Input: part model. Units: mm. Frame: model coordinates. Give positions to 0.01 mm unless a question says otherwise; leave off trailing zeros. Order: outer loops, then holes, each group sorted by start corner. A loop starts at its lowest first (then second) coordinate and runs counter-clockwise, first axis right, second up. Notation, with made-up numbers: (23.25, 57.25) - (59.25, 57.25) arc R31 ccw to (59.25, 94.25) - close; hole circle Ø8 at (5, 19). An arc over 180 degrees is marked (long way). Answer in a Markdown table with one row per item. Add a question column.
1. Ray query, line 1 (Z direction, x = -90.5, y = 2.7); line 2 (X direction, y = 2.1, z = 195); line 3 (Z direction, x = -74.5, y = 2.8). Return the intervals inside material, ascending. Write a range as [from, to].
2. Section query B-B on x = -109. Return loops of the section in (y, z) (3 decimals), and give its area (4 significant figures).
3. Contact query for flat-ended pins moving along their axis: pin 1 (2.5 mm diameter, centred on x = 39.5, z = -16.5, fed in from +Y); pin 2 (1 mm diameter, centred on y = 1, z = 45, fed in from -X); pin 3 (1.2 mm diameter, centred on x = -126.5, y = 1.5, fed in from +Z); pin 4 (1 mm diameter, centred on x = 36.5, z = 103.5, fed in from -Y). Output: stop coordinate, or through.
4. Section query C-C on x = -44. Return loops of the section in (y, z) (3 decimals).
5. Section query A-A on z = 195. Return loops of the section in (x, y).
6. Section query D-D on y = 1.9. Count the separate pieces of the cut face and the enclosed holes in it, and give its area (3 significant figures).
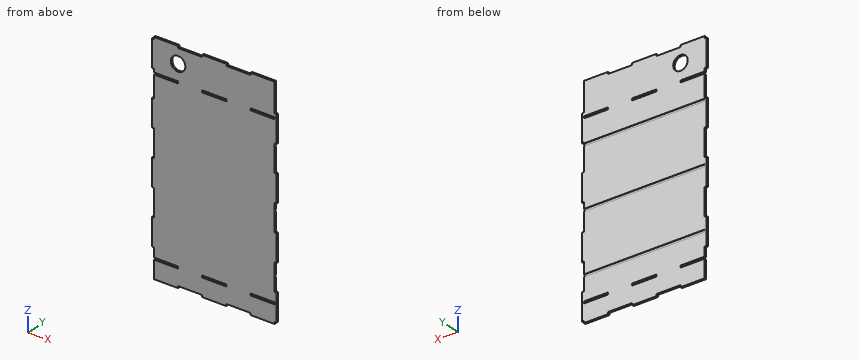
Autodesk Inventor part; units mm, degrees
ref_plane "YZ Plane" through (0, 0, 0) normal (1, 0, 0) x (0, 1, 0)
ref_plane "XZ Plane" through (0, 0, 0) normal (0, 1, 0) x (-1, 0, 0)
ref_plane "XY Plane" through (0, 0, 0) normal (0, 0, 1) x (1, 0, 0)
sketch "Sketch1" plane through (0, 0, 0) normal (0, 1, 0) x (-1, 0, 0)
  line L0 (-125, 225) -> (125, 225) construction
  line L1 (125, 225) -> (125, -225) construction
  line L2 (125, -225) -> (-125, -225) construction
  line L3 (-125, -225) -> (-125, 225) construction
  line L4 (-125, 225) -> (125, -225) construction
  line L5 (125, 225) -> (-125, -225) construction
  line L6 (125, 225) -> (75, 225) construction
  line L7 (75, 225) -> (75, 229)
  line L8 (75, 229) -> (125, 229)
  line L9 (125, 229) -> (125, 225)
  line L10 (125, 225) -> (129, 225)
  line L11 (129, 225) -> (129, 168.75)
  line L12 (129, 168.75) -> (125, 168.75)
  line L13 (125, 168.75) -> (125, 225) construction
  line L14 (-125, 225) -> (-129, 225) construction
  line L15 (-129, 225) -> (-129, 168.75) construction
  line L16 (-129, 168.75) -> (-125, 168.75)
  line L17 (-125, 168.75) -> (-125, 225)
  line L18 (125, -225) -> (75, -225) construction
  line L19 (75, -225) -> (75, -229)
  line L20 (75, -229) -> (125, -229)
  line L21 (125, -229) -> (125, -225)
  line L22 (125, 112.5) -> (125, 168.75)
  line L23 (125, 168.75) -> (129, 168.75)
  line L24 (129, 112.5) -> (125, 112.5)
  line L25 (129, 168.75) -> (129, 112.5) construction
  line L26 (-125, 112.5) -> (-125, 168.75) construction
  line L27 (-125, 168.75) -> (-129, 168.75)
  line L28 (-129, 168.75) -> (-129, 112.5)
  line L29 (-129, 112.5) -> (-125, 112.5)
  line L30 (125, 56.25) -> (125, 112.5) construction
  line L31 (125, 112.5) -> (129, 112.5)
  line L32 (129, 56.25) -> (125, 56.25)
  line L33 (129, 112.5) -> (129, 56.25)
  line L34 (-125, 56.25) -> (-125, 112.5)
  line L35 (-125, 112.5) -> (-129, 112.5)
  line L36 (-129, 112.5) -> (-129, 56.25) construction
  line L37 (-129, 56.25) -> (-125, 56.25)
  line L38 (125, 0) -> (125, 56.25)
  line L39 (125, 56.25) -> (129, 56.25)
  line L40 (129, 0) -> (125, 0)
  line L41 (129, 56.25) -> (129, 0) construction
  line L42 (-125, 0) -> (-125, 56.25) construction
  line L43 (-125, 56.25) -> (-129, 56.25)
  line L44 (-129, 56.25) -> (-129, 0)
  line L45 (-129, 0) -> (-125, 0)
  line L46 (125, -56.25) -> (125, 0) construction
  line L47 (125, 0) -> (129, 0)
  line L48 (129, -56.25) -> (125, -56.25)
  line L49 (129, 0) -> (129, -56.25)
  line L50 (-125, -56.25) -> (-125, 0)
  line L51 (-125, 0) -> (-129, 0)
  line L52 (-129, 0) -> (-129, -56.25) construction
  line L53 (-129, -56.25) -> (-125, -56.25)
  line L54 (125, -112.5) -> (125, -56.25)
  line L55 (125, -56.25) -> (129, -56.25)
  line L56 (129, -112.5) -> (125, -112.5)
  line L57 (129, -56.25) -> (129, -112.5) construction
  line L58 (-125, -112.5) -> (-125, -56.25) construction
  line L59 (-125, -56.25) -> (-129, -56.25)
  line L60 (-129, -56.25) -> (-129, -112.5)
  line L61 (-129, -112.5) -> (-125, -112.5)
  line L62 (125, -168.75) -> (125, -112.5) construction
  line L63 (125, -112.5) -> (129, -112.5)
  line L64 (129, -168.75) -> (125, -168.75)
  line L65 (129, -112.5) -> (129, -168.75)
  line L66 (-125, -168.75) -> (-125, -112.5)
  line L67 (-125, -112.5) -> (-129, -112.5)
  line L68 (-129, -112.5) -> (-129, -168.75) construction
  line L69 (-129, -168.75) -> (-125, -168.75)
  line L70 (125, -225) -> (125, -168.75)
  line L71 (125, -168.75) -> (129, -168.75)
  line L72 (129, -225) -> (125, -225) construction
  line L73 (129, -168.75) -> (129, -225) construction
  line L74 (-125, -225) -> (-125, -168.75) construction
  line L75 (-125, -168.75) -> (-129, -168.75)
  line L76 (-129, -168.75) -> (-129, -225)
  line L77 (-129, -225) -> (-125, -225)
  line L78 (75, 229) -> (75, 225)
  line L79 (25, 225) -> (25, 229)
  line L80 (25, 229) -> (75, 229) construction
  line L81 (75, 225) -> (25, 225)
  line L82 (75, -225) -> (25, -225)
  line L83 (25, -225) -> (25, -229)
  line L84 (25, -229) -> (75, -229) construction
  line L85 (75, -229) -> (75, -225)
  line L86 (25, 229) -> (25, 225)
  line L87 (-25, 225) -> (-25, 229)
  line L88 (-25, 229) -> (25, 229)
  line L89 (25, 225) -> (-25, 225) construction
  line L90 (25, -225) -> (-25, -225) construction
  line L91 (-25, -225) -> (-25, -229)
  line L92 (-25, -229) -> (25, -229)
  line L93 (25, -229) -> (25, -225)
  line L94 (-25, 229) -> (-25, 225)
  line L95 (-75, 225) -> (-75, 229)
  line L96 (-75, 229) -> (-25, 229) construction
  line L97 (-25, 225) -> (-75, 225)
  line L98 (-25, -225) -> (-75, -225)
  line L99 (-75, -225) -> (-75, -229)
  line L100 (-75, -229) -> (-25, -229) construction
  line L101 (-25, -229) -> (-25, -225)
  line L102 (-75, 229) -> (-75, 225)
  line L103 (-125, 225) -> (-125, 229)
  line L104 (-125, 229) -> (-75, 229)
  line L105 (-75, 225) -> (-125, 225) construction
  line L106 (-75, -225) -> (-125, -225) construction
  line L107 (-125, -225) -> (-125, -229)
  line L108 (-125, -229) -> (-75, -229)
  line L109 (-75, -229) -> (-75, -225)
  point P0 (0, 0)
  point P1 (75, -225)
  point P2 (25, -225)
  point P3 (-25, -225)
  point P4 (-75, -225)
  point P5 (-129, 168.75)
  point P6 (-129, 56.25)
  point P7 (-129, -56.25)
  point P8 (-129, -168.75)
  point P9 (-125, -225)
  point P10 (-25, -225)
  point P11 (75, -225)
  point P12 (125, -56.25)
  point P13 (125, 56.25)
  point P14 (125, 168.75)
  dimension "d0" = 250
  dimension "d1" = 450
  dimension "d2" = 50
  dimension "d3" = 4
  dimension "d4" = 4
  dimension "d5" = 56.25
  dimension "d6" = 4
  dimension "d7" = 56.25
  dimension "d8" = 50
  dimension "d9" = 4
  dimension "d12" = 56.25
  dimension "d19" = 50
extrude "Extrusion1" add sketch "Sketch1" along normal blind 4
sketch "Sketch3" plane through (0, 4, 0) normal (0, 1, 0) x (1, 0, 0)
  line L0 (-129, 56.25) -> (-129, 0)
  line L1 (-129, 15.625) -> (125, 15.625) construction
  line L2 (125, 0) -> (125, 56.25)
  line L3 (-129, 13.125) -> (125, 13.125)
  line L4 (125, 13.125) -> (125, 18.125)
  line L5 (125, 18.125) -> (-129, 18.125)
  line L6 (-129, 18.125) -> (-129, 13.125)
  line L7 (-129, 18.125) -> (-125, 18.125)
  line L8 (-125, 18.125) -> (-125, 13.125)
  line L9 (-125, 13.125) -> (-129, 13.125)
  line L10 (-129, 13.125) -> (-129, 18.125)
  line L11 (-25, -225) -> (-25, -229)
  line L12 (-25, -229) -> (25, -229)
  line L13 (25, -229) -> (25, -225)
  line L14 (25, -225) -> (75, -225)
  line L15 (75, -225) -> (75, -229)
  line L16 (75, -229) -> (125, -229)
  line L17 (125, -229) -> (125, -168.75)
  line L18 (125, -168.75) -> (129, -168.75)
  line L19 (129, -168.75) -> (129, -112.5)
  line L20 (129, -112.5) -> (125, -112.5)
  line L21 (125, -112.5) -> (125, -56.25)
  line L22 (125, -56.25) -> (129, -56.25)
  line L23 (129, -56.25) -> (129, 0)
  line L24 (129, 0) -> (125, 0)
  line L25 (125, 0) -> (125, 56.25)
  line L26 (125, 56.25) -> (129, 56.25)
  line L27 (129, 56.25) -> (129, 112.5)
  line L28 (129, 112.5) -> (125, 112.5)
  line L29 (125, 112.5) -> (125, 168.75)
  line L30 (125, 168.75) -> (129, 168.75)
  line L31 (129, 168.75) -> (129, 225)
  line L32 (129, 225) -> (125, 225)
  line L33 (125, 225) -> (125, 229)
  line L34 (125, 229) -> (75, 229)
  line L35 (75, 229) -> (75, 225)
  line L36 (75, 225) -> (25, 225)
  line L37 (25, 225) -> (25, 229)
  line L38 (25, 229) -> (-25, 229)
  line L39 (-25, 229) -> (-25, 225)
  line L40 (-25, 225) -> (-75, 225)
  line L41 (-75, 225) -> (-75, 229)
  line L42 (-75, 229) -> (-125, 229)
  line L43 (-125, 229) -> (-125, 168.75)
  line L44 (-125, 168.75) -> (-129, 168.75)
  line L45 (-129, 168.75) -> (-129, 112.5)
  line L46 (-129, 112.5) -> (-125, 112.5)
  line L47 (-125, 112.5) -> (-125, 56.25)
  line L48 (-125, 56.25) -> (-129, 56.25)
  line L49 (-129, 56.25) -> (-129, 0)
  line L50 (-129, 0) -> (-125, 0)
  line L51 (-125, 0) -> (-125, -56.25)
  line L52 (-125, -56.25) -> (-129, -56.25)
  line L53 (-129, -56.25) -> (-129, -112.5)
  line L54 (-129, -112.5) -> (-125, -112.5)
  line L55 (-125, -112.5) -> (-125, -168.75)
  line L56 (-125, -168.75) -> (-129, -168.75)
  line L57 (-129, -168.75) -> (-129, -225)
  line L58 (-129, -225) -> (-125, -225)
  line L59 (-125, -225) -> (-125, -229)
  line L60 (-125, -229) -> (-75, -229)
  line L61 (-75, -229) -> (-75, -225)
  line L62 (-75, -225) -> (-25, -225)
  line L63 (-125, -112.5) -> (-125, -168.75)
  line L64 (-109.8402, -80.4521) -> (129, -140.625) construction
  line L65 (129, -168.75) -> (129, -112.5)
  line L66 (-125, -110.625) -> (125, -110.625)
  line L67 (125, -110.625) -> (125, -105.625)
  line L68 (125, -105.625) -> (-125, -105.625)
  line L69 (-125, -105.625) -> (-125, -110.625)
  line L70 (-125, -110.625) -> (125, -105.625) construction
  line L71 (125, -110.625) -> (-125, -105.625) construction
  line L72 (125, 0) -> (125, 56.25)
  line L73 (-125, 0) -> (-125, -56.25)
  line L74 (129, 168.75) -> (129, 225)
  line L75 (129, 139.375) -> (-125, 139.375) construction
  line L76 (-125, 136.875) -> (125, 136.875)
  line L77 (125, 136.875) -> (125, 141.875)
  line L78 (125, 141.875) -> (-125, 141.875)
  line L79 (-125, 141.875) -> (-125, 136.875)
  line L80 (-125, 136.875) -> (125, 141.875) construction
  line L81 (125, 136.875) -> (-125, 141.875) construction
  line L82 (-125, 229) -> (-125, 168.75)
  line L83 (125, 112.5) -> (125, 168.75)
  point P0 (0, 0)
  point P1 (-129, 18.125)
  point P2 (-125, 18.125)
  point P3 (-125, 13.125)
  point P4 (0, -108.125)
  point P5 (-125, -138.125)
  point P6 (-125, -143.125)
  point P7 (0, 139.375)
  point P8 (-125, 199.375)
  point P9 (-125, 194.375)
  dimension "d30" = 5
  dimension "d34" = 5
  dimension "d35" = 5
  dimension "d36" = 5
  dimension "d56" = 118.375
  dimension "d57" = 118.75
  dimension "d59" = 118.75
extrude "Extrusion2" cut sketch "Sketch3" against normal blind 1 contours L5 L2 L3 L8 | L76 L79 L78 L29 | L21 L66 L69 L68
sketch "Sketch4" plane through (0, 4, 0) normal (0, 1, 0) x (1, 0, 0)
  line L0 (-125, -158) -> (-75, -158)
  line L1 (-75, -158) -> (-75, -162)
  line L2 (-75, -162) -> (-125, -162)
  line L3 (-125, -162) -> (-125, -158)
  line L4 (-75, -225) -> (-25, -225)
  line L5 (125, -110.625) -> (-125, -110.625)
  line L6 (-75, -158) -> (-25, -158)
  line L7 (-25, -158) -> (-25, -162)
  line L8 (-25, -162) -> (-75, -162)
  line L9 (-75, -162) -> (-75, -158)
  line L10 (-25, -158) -> (25, -158)
  line L11 (25, -158) -> (25, -162)
  line L12 (25, -162) -> (-25, -162)
  line L13 (-25, -162) -> (-25, -158)
  line L14 (25, -158) -> (75, -158)
  line L15 (75, -158) -> (75, -162)
  line L16 (75, -162) -> (25, -162)
  line L17 (25, -162) -> (25, -158)
  line L18 (75, -158) -> (125, -158)
  line L19 (125, -158) -> (125, -162)
  line L20 (125, -162) -> (75, -162)
  line L21 (75, -162) -> (75, -158)
  line L22 (-125, 0) -> (-125, -56.25)
  line L23 (-125, 192) -> (-75, 192)
  line L24 (-75, 192) -> (-75, 188)
  line L25 (-75, 188) -> (-125, 188)
  line L26 (-125, 188) -> (-125, 192)
  line L27 (-75, 192) -> (-25, 192)
  line L28 (-25, 192) -> (-25, 188)
  line L29 (-25, 188) -> (-25, 192)
  line L30 (-25, 188) -> (-75, 188)
  line L31 (-75, 188) -> (-75, 192)
  line L32 (-25, 192) -> (25, 192)
  line L33 (25, 188) -> (-25, 188)
  line L34 (25, 192) -> (25, 188)
  line L35 (25, 188) -> (25, 192)
  line L36 (25, 192) -> (75, 192)
  line L37 (75, 192) -> (75, 188)
  line L38 (75, 188) -> (75, 192)
  line L39 (75, 192) -> (125, 192)
  line L40 (125, 192) -> (125, 188)
  line L41 (125, 188) -> (75, 188)
  line L42 (75, 188) -> (25, 188)
  point P0 (0, 0)
  point P1 (-125, -160)
  point P2 (-75, -160)
  point P3 (-25, -160)
  point P4 (25, -160)
  point P5 (75, -160)
  point P6 (-25, -162)
  point P7 (-125, 190)
  point P8 (-25, 190)
  point P9 (-75, 190)
  point P10 (25, 190)
  point P11 (75, 190)
  point P12 (-25, 188)
  point P13 (-125, -168.75)
  dimension "d37" = 50
  dimension "d38" = 4
  dimension "d39" = 63
  dimension "d42" = 50
  dimension "d51" = 350
extrude "Extrusion3" cut sketch "Sketch4" against normal up to next contours L0 L1 L2 L3 | L10 L11 L12 L7 | L18 L19 L20 L15 | L23 L24 L25 L26 | L32 L34 L33 L28 | L39 L40 L41 L37
sketch "Sketch6" plane through (0, 4, 0) normal (0, 1, 0) x (1, 0, 0)
  circle A0 centre (-75, -195) radius 15
  line L0 (-75, -225) -> (-25, -225)
  line L1 (-125, -162) -> (-125, -168.75)
  point P0 (0, 0)
  point P1 (-125, -165.375)
  dimension "d60" = 30
  dimension "d61" = 30
  dimension "d62" = 50
extrude "Extrusion4" cut sketch "Sketch6" against normal through all
properties part number "Rear_V2"
Answer:
| question | item | result |
|---|---|---|
| 1 | line 1 | z = [-229, -192], [-188, 158], [162, 229] |
| 1 | line 2 | x = [-129, -90], [-60, 125] |
| 1 | line 3 | z = [-225, 180.01], [209.99, 225] |
| 2 | outline | (0, -229) - (4, -229) - (4, -192) - (0, -192) - close; (0, -188) - (4, -188) - (4, -141.875) - (3, -141.875) - (3, -136.875) - (4, -136.875) - (4, -18.125) - (3, -18.125) - (3, -13.125) - (4, -13.125) - (4, 105.625) - (3, 105.625) - (3, 110.625) - (4, 110.625) - (4, 158) - (0, 158) - close; (0, 162) - (4, 162) - (4, 229) - (0, 229) - close |
| 2 | area | 1,785 mm² |
| 3 | pin 1 | stops at y = 3 |
| 3 | pin 2 | stops at x = -125 |
| 3 | pin 3 | stops at z = 225 |
| 3 | pin 4 | stops at y = 0 |
| 4 | outline | (0, -225) - (4, -225) - (4, -141.875) - (3, -141.875) - (3, -136.875) - (4, -136.875) - (4, -18.125) - (3, -18.125) - (3, -13.125) - (4, -13.125) - (4, 105.625) - (3, 105.625) - (3, 110.625) - (4, 110.625) - (4, 225) - (0, 225) - close |
| 5 | outline | (-129, 0) - (-90, 0) - (-90, 4) - (-129, 4) - close; (-60, 0) - (125, 0) - (125, 4) - (-60, 4) - close |
| 6 | separate pieces | 1 |
| 6 | enclosed holes | 5 |
| 6 | area | 114,000 mm² |
